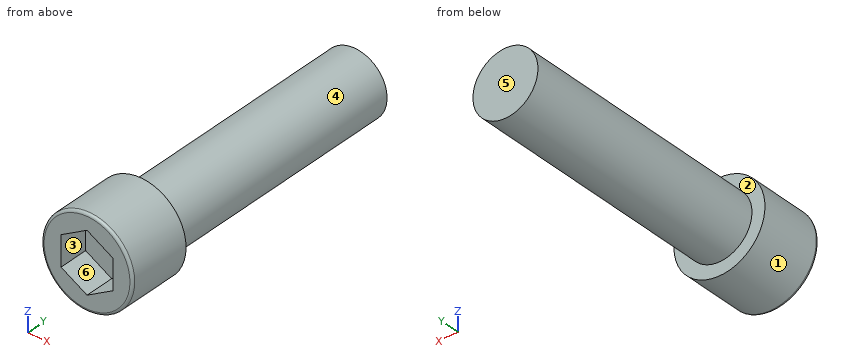
Solid Edge part; units mm, degrees
sketch "Sketch1" plane through (0, 0, 0) normal (0, -1, 0) x (1, 0, 0)
  circle A0 centre (0, 0) radius 3.5
extrude "Protrusion1" add sketch "Sketch1" against normal blind 5
sketch "Sketch2" plane through (0, 5, 0) normal (0, 1, 0) x (-1, 0, 0)
  circle A0 centre (0, 0) radius 2.5
extrude "ExtrudedProtrusion_2" add sketch "Sketch2" along normal blind 20
fillet "Round_1" radius 0.2 1 edges at (-3.5, 0, 0)
sketch "Sketch3" plane through (0, 0, 0) normal (0, -1, 0) x (1, 0, 0)
  line L0 (0, 2.3094) -> (-2, 1.1547)
  line L1 (-2, 1.1547) -> (-2, -1.1547)
  line L2 (-2, -1.1547) -> (0, -2.3094)
  line L3 (0, -2.3094) -> (2, -1.1547)
  line L4 (2, -1.1547) -> (2, 1.1547)
  line L5 (2, 1.1547) -> (0, 2.3094)
extrude "ExtrudedCutout_2" cut sketch "Sketch3" against normal blind 2.3
properties material "Steel"
Geometry check sheet. Reference: the model listing, model coordinates, mm. Face numbers are marked on the shaded views. A direction names the side the tool comes from. Coordinates: 2 decimals unless noted, no trailing zeros. Order: outer loops, then holes, each group sorted by start corner. A loop starts at its lowest first (then second) coordinate and runs counter-clockwise, first axis right, second up.
Item 1: Section check A-A (z = 0). Enter the section's corners in (x, y), plus the area to 3 significant figures.
Item 2: Mould release check, pull along X, two halves, no side actions. Record for the marked faces 1, 2 and 3: released by +X, released by -X, zero draft, split by the parting line, or undercut.
Item 3: Depth check by flat-ended pin: pin 1 (1.5 mm diameter, centred on y = 18.5, z = 0, fed in from +X); pin 2 (2 mm diameter, centred on x = 0.5, z = 0, fed in from -Y); pin 3 (3 mm diameter, centred on y = 5, z = -2.5, fed in from -X). Enter the tip coordinate at first touch or a pass-through.
Item 4: Tool access check on the marked faces 4, 5 and 6. Record the directions out of +Z, -Z, +X, -X, +Y, -Y that give a thin tool (end or side, any length) a straight path to the whole face; none if there is none.
Item 5: Scan lines: line 1 along Y through (x, z) = (1.75, 0.5); line 2 along Y through (x, z) = (0.25, 3); line 3 along Z through (x, y) = (-1.5, 9). Record each from-to range of solid material in increasing order.
Item 6: Section check B-B (y = 23.25). Enter the section's corners in (x, z).
Check sheet entries:
1. outline: (-3.5, 0.2) arc R0.2 ccw to (-3.3, 0) - (-2, 0) - (-2, 2.3) - (2, 2.3) - (2, 0) - (3.3, 0) arc R0.2 ccw to (3.5, 0.2) - (3.5, 5) - (2.5, 5) - (2.5, 25) - (-2.5, 25) - (-2.5, 5) - (-3.5, 5) - close
1. area: 126 mm2
2. face 1: split by the parting line
2. face 2: zero draft
2. face 3: undercut
3. pin 1: stops at x = 2.5
3. pin 2: stops at y = 2.3
3. pin 3: stops at x = -3.35
4. face 4: +Y
4. face 5: +Z, -Z, +X, -X, +Y
4. face 6: -Y
5. line 1: y = 2.3 to 25
5. line 2: y = 0 to 5
5. line 3: z = -2 to 2
6. outline: circle Ø5 at (0, 0)
